CAD build for the part. Positions are in the model's coordinates, mm. Face numbers are marked on the shaded views. Round coordinates to 2 decimals unless told otherwise and drop trailing zeros. Order: outer loops, then holes, each group sorted by start corner. A loop starts at its lowest first (then second) coordinate and runs counter-clockwise, first axis right, second up. Notation, with made-up numbers: (41.25, 19) -> (67.25, 19) arc R10 cw to (67.25, 24) -> close; hole circle Ø1 at (55, -9.75). An arc over 180 degrees is marked (long way). Return JSON: item names as keys, results as strings. Group by question number.
Q1. Mould opens along X. For the marked faces 1, 2 and 3 say: +X half, -X half, draft (parallel to the pull), parting line (faces both ways), or undercut.
Q2. Probe line 1 along Y through (x, z) = (81, -32.5); line 2 along X through (y, z) = (7.5, -23); line 3 along Z through (x, y) = (48, -8.25). List the from-to ranges inside material, lowest first.
Q3. Cut at B-B (x = 49). Write the cut outline in (y, z), then the cut area to 3 significant figures.
Q4. Cut at D-D (z = -42). Write the cut outline in (x, y), then the cut area to 3 significant figures.
Q5. Flat gauge pins, fed straight in: pin 1 (2 mm diameter, centred on x = 51.5, y = 8.5, fed in from -Z); pin 2 (4 mm diameter, centred on x = 41.5, y = -7, fed in from -Z); pin 3 (2 mm diameter, centred on x = 28, y = 1, fed in from +Z). Where does each tip first touch, or does it go through?
Q6. Cut at A-A (z = -9). Write the cut outline in (x, y).
Q7. Cut at C-C (y = 1). Write the cut outline in (x, z), then the cut area to 3 significant figures.
from build123d import *

# Parameters (mm, degrees)
REVOLVE1_ANGLE     = 180
SKETCH2_R          = 1.5
CUT_EXTRUDE1_DEPTH = 21


with BuildPart() as part:
    # Sketch1 → Revolve1 (revolve)
    with BuildSketch(Plane.XY):
        Polygon((-4.971917279, -11.985029192), (4.445516801, -11.985029192), (4.445516801, -9.102141208), (-0.167103973, -9.102141208), (-0.167103973, 10.117112016), (4.445516801, 10.117112016), (4.445516801, 13), (-4.971917279, 13), align=None)
    revolve(axis=Axis((48.841991749, -11.985029192, 0), (0, -1, 0)), revolution_arc=REVOLVE1_ANGLE)

    # Sketch2 → Cut-Extrude1 (cut)
    with BuildSketch(Plane.XY.offset(-54)):
        with Locations(Location((45.028082721, 1, 0), (0, 0, 180))):
            Circle(SKETCH2_R)
    extrude(amount=CUT_EXTRUDE1_DEPTH, mode=Mode.SUBTRACT)


solid = part.part
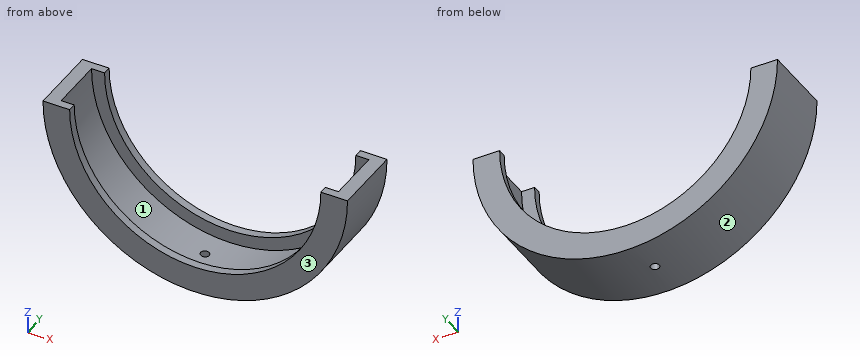
Solution:
{
 "1": {"face 1": "undercut", "face 2": "parting line", "face 3": "draft"},
 "2": {"line 1": "y = -11.99 to -9.1, 10.12 to 13", "line 2": "x = 0.19 to 5.57, 92.12 to 97.49", "line 3": "z = -53.81 to -49"},
 "3": {"outline": "(-11.99, -53.81) -> (13, -53.81) -> (13, -44.4) -> (10.12, -44.4) -> (10.12, -49.01) -> (-9.1, -49.01) -> (-9.1, -44.4) -> (-11.99, -44.4) -> close", "area": "147 mm²"},
 "4": {"outline": "(15.2, -11.99) -> (34.45, -11.99) -> (34.45, -9.1) -> (23.59, -9.1) -> (23.59, 10.12) -> (34.45, 10.12) -> (34.45, 13) -> (15.2, 13) -> close; (63.23, -11.99) -> (82.49, -11.99) -> (82.49, 13) -> (63.23, 13) -> (63.23, 10.12) -> (74.1, 10.12) -> (74.1, -9.1) -> (63.23, -9.1) -> close", "area": "544 mm²"},
 "5": {"pin 1": "stops at z = -53.79", "pin 2": "stops at z = -53.55", "pin 3": "stops at z = -43.87"},
 "6": {"outline": "(-4.21, -11.99) -> (5.37, -11.99) -> (5.37, -9.1) -> (0.67, -9.1) -> (0.67, 10.12) -> (5.37, 10.12) -> (5.37, 13) -> (-4.21, 13) -> close; (92.32, -11.99) -> (101.9, -11.99) -> (101.9, 13) -> (92.32, 13) -> (92.32, 10.12) -> (97.02, 10.12) -> (97.02, -9.1) -> (92.32, -9.1) -> close"},
 "7": {"outline": "(-4.97, 0) arc R53.81 ccw to (43.53, -53.55) -> (43.53, -48.72) arc R49.01 cw to (-0.17, 0) -> close; (46.53, -53.76) arc R53.81 ccw to (102.66, 0) -> (97.85, 0) arc R49.01 cw to (46.53, -48.95) -> close", "area": "762 mm²"}
}
